Check sheet for the drawn part. Datum: minimum x, y, z corner. Units: mm. Round coordinates to 2 decimals unless told otherwise and drop trailing zeros. Order: outer loops, then holes, each group sorted by start corner. A loop starts at its lowest first (then second) coordinate and runs counter-clockwise, first axis right, second up. Notation, with made-up numbers: (74.25, 46.25) -> (86.25, 46.25) arc R23 cw to (86.25, 71.25) -> close; hole circle Ø7 at (-10.5, 14.5). An arc over 180 degrees is marked (long way). Answer in a Markdown table with one row per item.
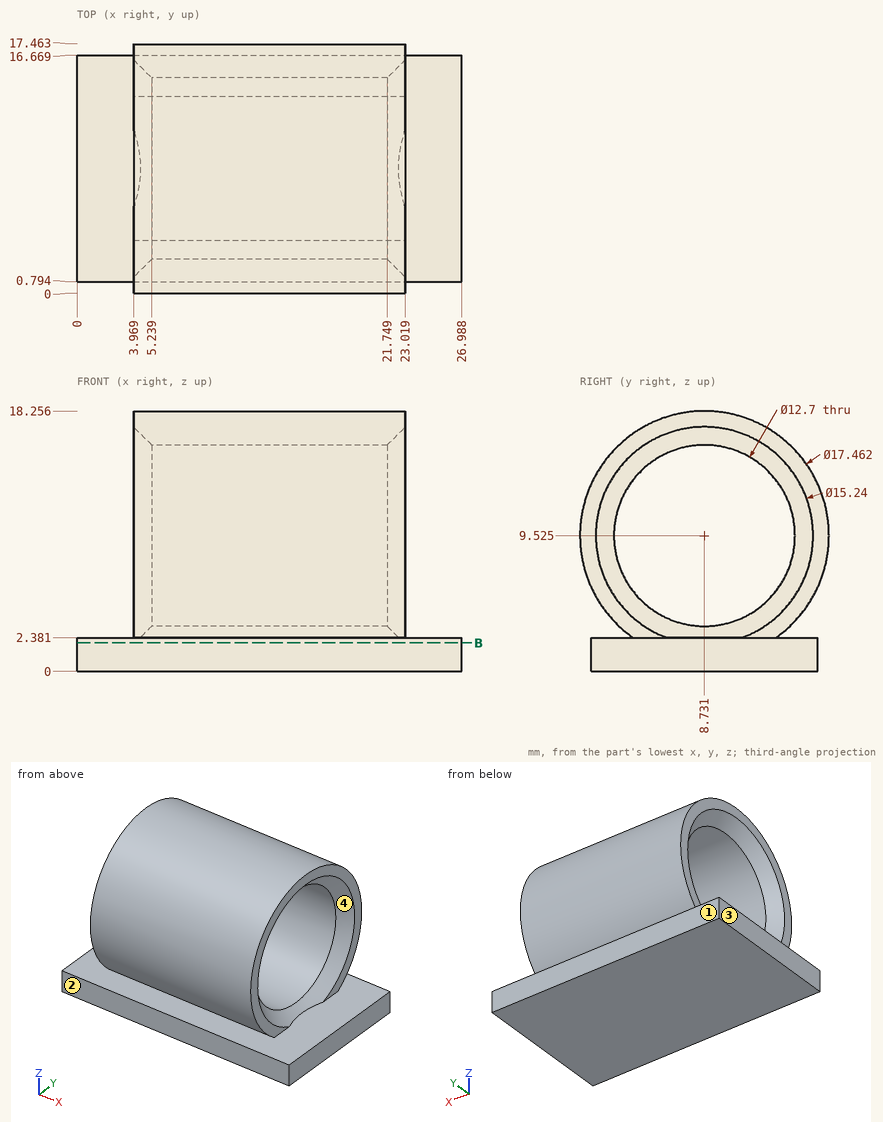
(1) Depth check by flat-ended pin: pin 1 Ø1.9 at (x, z) = (19.5, 1.5) entering from -Y; pin 2 Ø5 at (y, z) = (10, 14) entering from +X; pin 3 Ø4 at (x, y) = (10.5, 2) entering from +Z. Enter the tip coordinate at first touch or a pass-through.
Solutions:
| item | result |
|---|---|
| pin 1 | y = 0.79 |
| pin 2 | x = 22.55 |
| pin 3 | z = 16.86 |
(2) Scan lines: probe 1 along Z at (x, y) = (18.25, 14.5) (1 decimal); probe 2 along Y at (x, z) = (14.25, 9.25) (1 decimal); probe 3 along Z at (x, y) = (9.75, 14) (1 decimal). Record each from-to range of solid material in increasing order. Write a range as from..to.
Solutions:
| item | result |
|---|---|
| probe 1 | 0..2.4, 3..6.9, 12.2..16.1 |
| probe 2 | 0..2.4, 15.1..17.5 |
| probe 3 | 0..2.4, 2.6..6, 13.1..16.5 |
(3) Draft check along Y on the marked faces 1, 2, 3 and 4. Enter one of: pulls with the +Y half, pulls with the -Y half, needs draft (parallel to the pull), parting line crosses it, or undercut.
Solutions:
| item | result |
|---|---|
| face 1 | pulls with the +Y half |
| face 2 | pulls with the -Y half |
| face 3 | needs draft |
| face 4 | undercut |
(4) Section check B-B on z = 2. Record the boundary of the cut face in (x, y).
Solutions:
| item | result |
|---|---|
| outline | (0, 0.79) -> (26.99, 0.79) -> (26.99, 16.67) -> (0, 16.67) -> close |
